Model file for the job. Use its own axes, mm. A direction names the side the tool comes from. Coordinates: 2 decimals unless noted, no trailing zeros. Loops run counter-clockwise (first coordinate to the right, second up) from the corner with the lowest first, then second, coordinate; pieces in that order, holes last.
from build123d import *

# Parameters (mm, degrees)
F0_R     = 12
F1_DEPTH = 15
F2_W     = 12
F2_H     = 85
F5_DEPTH = 15
F6_W     = 22
F6_H     = 2
F6_H_2   = 15
F7_DEPTH = 25.4


with BuildPart() as f1:
    # F0 (on Top) → F1 (new body, symmetric)
    with BuildSketch(Plane.XY):
        Circle(F0_R)
    extrude(amount=F1_DEPTH, both=True)

    # F2 (on Right) → F3 (revolve)
    with BuildSketch(Plane.YZ):
        with Locations((6, 57.5)):
            Rectangle(F2_W, F2_H)
        with BuildLine():
            Line((12, 100), (12, 15))
            add(Edge.make_bspline(
                [(15, 50), (14.8483760761, 36.7983569986), (13.4529237629, 24.5626545335), (12, 15)],
                knots=[0.5442355016, 0.5442355016, 0.5442355016, 0.5442355016, 1, 1, 1, 1], degree=3))
            Line((15, 50), (15, 55.0494137852))
            add(Edge.make_bspline(
                [(12, 100), (13.4204155957, 84.714924594), (14.8440376845, 69.3918255439), (15, 55.0494137852)],
                knots=[0, 0, 0, 0, 0.4866410928, 0.4866410928, 0.4866410928, 0.4866410928], degree=3))
        make_face()
        with BuildLine():
            Line((15, 55.0494137852), (15, 50))
            add(Edge.make_bspline(
                [(15, 55.0494137852), (15.0184582796, 53.3519765173), (15.019160532, 51.6682756719), (15, 50)],
                knots=[0.4866410928, 0.4866410928, 0.4866410928, 0.4866410928, 0.5442355016, 0.5442355016, 0.5442355016, 0.5442355016], degree=3))
        make_face()
    revolve(axis=Axis((0, 0, 50), (0, 0, -1)))

    # F4 (on Right) → F5 (join, symmetric)
    with BuildSketch(Plane.YZ):
        with BuildLine():
            Line((-12, 100), (12, 100))
            Line((12, 100), (12, 140))
            ThreePointArc((12, 140), (0, 128), (-12, 140))
            Line((-12, 140), (-12, 100))
        make_face()
        with BuildLine():
            ThreePointArc((-12, 140), (0, 128), (12, 140))
            Line((12, 140), (7.5, 140))
            ThreePointArc((7.5, 140), (0, 132.5), (-7.5, 140))
            Line((-7.5, 140), (-12, 140))
        make_face()
        with BuildLine():
            Line((7.5, 140), (12, 140))
            ThreePointArc((12, 140), (0, 152), (-12, 140))
            Line((-12, 140), (-7.5, 140))
            ThreePointArc((-7.5, 140), (0, 147.5), (7.5, 140))
        make_face()
    extrude(amount=F5_DEPTH, both=True)

    # F6 (on face) → F7 (cut)
    with BuildSketch(Plane(origin=(0, 12, 0), x_dir=(-1, 0, 0), z_dir=(0, 1, 0))):
        with Locations((0, 156)):
            Rectangle(F6_W, F6_H)
        with BuildLine():
            add(Edge.make_bspline(
                [(0, 123), (3.6666666667, 123), (7.3333333333, 124), (11, 125)],
                knots=[0.5, 0.5, 0.5, 0.5, 1, 1, 1, 1], degree=3))
            Line((11, 125), (-11, 125))
            add(Edge.make_bspline(
                [(-11, 125), (-7.3333333333, 124), (-3.6666666667, 123), (0, 123)],
                knots=[0, 0, 0, 0, 0.5, 0.5, 0.5, 0.5], degree=3))
        make_face()
        with Locations((0, 147.5)):
            Rectangle(F6_W, F6_H_2)
        with Locations((0, 132.5)):
            Rectangle(F6_W, F6_H_2)
    extrude(amount=-F7_DEPTH, mode=Mode.SUBTRACT)


solid = f1.part
Q1. Mould opens along Z. For faces 1 (the cylindrical face through (13.028, 0.976, 147.436)), 2 (the flat face through (0, -12, 116)), 3 (the cylindrical face through (-13, 0, 152)) say: +Z half, -Z half, draft (parallel to the pull), parting line (faces both ways), or undercut.
Answers:
face 1: undercut
face 2: draft
face 3: +Z half
Q2. Slice it at A-A (y = 0). Count the separate pieces of the cut face and the enclosed holes in it, and give its area (3 significant figures).
Answers:
separate pieces: 3
enclosed holes: 0
area: 3,900 mm2
Q3. Slice it at B-B (z = 8.5). List the corners of the cut face in (x, y), and give its area (3 significant figures).
Answers:
outline: circle Ø24 at (0, 0)
area: 452 mm2
Q4. Flat gauge pins, fed straight in: P1, Ø5, axis at x = 9.5, z = 112, coming from the +Y side; P2, Ø1.5, axis at x = 10, y = -4, coming from the +Z side; P3, Ø1.5, axis at x = 11, z = 43.5, coming from the -Y side; P4, Ø13.5, axis at y = 0, z = 140, coming from the +X side. Where does each tip first touch, or does it go through?
Answers:
P1: stops at y = 12
P2: stops at z = 124.93
P3: stops at y = -10.71
P4: passes through
Q5. Which spindle directions (+Z, -Z, +X, -X, +Y, -Y) get a long thin tool onto all of the face, cutting with end or side? Do faces 4 (the cylindrical face through (-11.99, 0.53, 0.21)), 5 (the flat face through (0, 12, 115)), 6 (the flat face through (-11, 0, 132)). Say none if no direction does.
Answers:
face 4: -Z
face 5: +Z, +X, -X, +Y
face 6: +Z, +Y, -Y
Q6. Drill centre lines: line 1 (Y direction, x = -12.8, z = 140); line 2 (X direction, y = -3, z = 125.5); line 3 (X direction, y = -9, z = 73.5). Where is each one in solid material? Low to high.
Answers:
line 1: y = -12 to -7.5, 7.5 to 12
line 2: x = -15 to -11, 11 to 15
line 3: x = -11.02 to 11.02
